Read the model definition and answer for the solid it produces. Units are mm, in the model's axes. A direction names the side the tool comes from. Give positions to 0.01 mm unless a question says otherwise; leave off trailing zeros. Write each loop counter-clockwise with the first axis right and the second up, starting at its lowest first coordinate (ties: lowest second). Pieces come first, ordered by that corner, then holes. Notation, with made-up numbers: M -13,-20.5 L -8,-20.5 A12 cw -8,-10.5 Z; hole C 47.5,81.25 d11. An arc over 180 degrees is marked long. Put each result on its own line as item: value.
from build123d import *

# Parameters (mm, degrees)
F0_W     = 355.6
F0_H     = 88.9
F1_DEPTH = 19.05
F2_W     = 355.6
F2_H     = 19.05
F3_DEPTH = 6.35
F4_R     = 5.08
F5_R     = 1.5875
F6_DEPTH = 19.051


with BuildPart() as f1:
    # F0 (on Right) → F1 (new body)
    with BuildSketch(Plane.YZ):
        with Locations((177.8, -44.45)):
            Rectangle(F0_W, F0_H)
    extrude(amount=-F1_DEPTH)

    # F2 (on Right) → F3 (cut)
    with BuildSketch(Plane.YZ):
        with Locations((177.8, -73.025)):
            Rectangle(F2_W, F2_H)
    extrude(amount=-F3_DEPTH, mode=Mode.SUBTRACT)

    # F4
    f4_edges = [f1.edges().sort_by_distance(p)[0] for p in [
        (-9.525, 0, 0),
    ]]
    fillet(f4_edges, radius=F4_R)

    # F5 (on Right) → F6 (cut, through all)
    with BuildSketch(Plane.YZ):
        with Locations((12.7, -73.025)):
            Circle(F5_R)
        with Locations((114.3, -73.025)):
            Circle(F5_R)
        with Locations((215.9, -73.025)):
            Circle(F5_R)
        with Locations((317.5, -73.025)):
            Circle(F5_R)
    extrude(amount=-F6_DEPTH, mode=Mode.SUBTRACT)


solid = f1.part
(1) Straight lines are drawn through the part: line 1 along Z through (x, y) = (-14.75, 215.9); line 2 along Z through (x, y) = (-5.25, 99); line 3 along X through (y, z) = (97.5, -77). For each, find the intervals that lie inside material, in ascending order. Write a range as from..to.
Result:
line 1: z = -88.9..-74.61, -71.44..0
line 2: z = -88.9..-82.55, -63.5..0
line 3: x = -19.05..-6.35
(2) Section A-A on x = -3 is taken. Determine the outline of the cut face in (y, z).
Result:
outline: M 0,-88.9 L 355.6,-88.9 L 355.6,-82.55 L 0,-82.55 Z; M 0,-63.5 L 355.6,-63.5 L 355.6,0 L 5.08,0 A5.08 ccw 0,-5.08 Z
(3) Which of the six approach directions +Z, -Z, +X, -X, +Y, -Y give full straight-line access (tool end or side, diameter ignored) to faces 5 (the face through (-6.35, 175, -73)), 6 (the face through (-19.05, 175, -44))?
Result:
face 5: +X, +Y, -Y
face 6: +Z, -Z, -X, +Y, -Y
(4) For a pull along Z with two mould halves and no side action, classify faces 1 (the face through (-9, 0, -48)), 2 (the face through (-3, 175, -82.55)), 3 (the face through (-9, 175, -88.9)), 4 (the face through (-3, 175, -63.5)) as +Z half, -Z half, draft (parallel to the pull), parting line (faces both ways), or undercut.
Result:
face 1: draft
face 2: undercut
face 3: -Z half
face 4: undercut
(5) Section B-B on y = 245.5 is taken. Determine the outline of the cut face in (x, z).
Result:
outline: M -19.05,-88.9 L 0,-88.9 L 0,-82.55 L -6.35,-82.55 L -6.35,-63.5 L 0,-63.5 L 0,0 L -19.05,0 Z
(6) Given pin 1 Ø15 at (y, z) = (138.5, -72.5) entering from +X, flat-ended and moving along its own axis, determine where the tip first touches the part or whether it passes through.
Result:
pin 1: stops at x = -6.35
